Autodesk Inventor part; units mm, degrees
ref_plane "YZ Plane" through (0, 0, 0) normal (1, 0, 0) x (0, 1, 0)
ref_plane "XZ Plane" through (0, 0, 0) normal (0, 1, 0) x (-1, 0, 0)
ref_plane "XY Plane" through (0, 0, 0) normal (0, 0, 1) x (1, 0, 0)
sketch "Sketch1" plane through (0, 0, 0) normal (0, 1, 0) x (-1, 0, 0)
  line L0 (13.2677, 19.6408) -> (-12.1323, 19.6408)
  line L1 (-12.1323, 19.6408) -> (-12.1323, -18.4592)
  line L2 (-12.1323, -18.4592) -> (13.2677, -18.4592)
  line L3 (13.2677, -18.4592) -> (13.2677, 19.6408)
  point P0 (0, 0)
  dimension "d0" = 25.4
  dimension "d1" = 38.1
extrude "Extrusion1" add sketch "Sketch1" along normal blind 3.175
hole "Hole1" at (-9.6799, 3.175, 14.8783) direction (0, -1, 0) diameter 4.4958 depth 3.175
hole "Hole2" at (8.5446, 3.175, 14.8783) direction (0, -1, 0) diameter 4.4958 depth 3.175
hole "Hole3" at (-9.6799, 3.175, -13.6967) direction (0, -1, 0) diameter 4.4958 depth 3.175
hole "Hole4" at (8.5446, 3.175, -13.6967) direction (0, -1, 0) diameter 4.4958 depth 3.175
hole "Hole5" at (-0.5677, 3.175, -6.5466) direction (0, -1, 0) diameter 2.54 depth 3.175
hole "Hole6" at (-0.5677, 3.175, 7.7345) direction (0, -1, 0) diameter 2.54 depth 3.175
sketch "Sketch2" plane through (0, 3.175, 0) normal (0, 1, 0) x (1, 0, 0)
  circle A0 centre (0, 0) radius 3.175
  dimension "d58" = 6.35
extrude "Extrusion2" add sketch "Sketch2" along normal blind 304.8
sketch "Sketch3" plane through (0, 0, 0) normal (1, 0, 0) x (0, 1, 0)
  point P0 (0, 0)
properties part number "rotatable rod table"
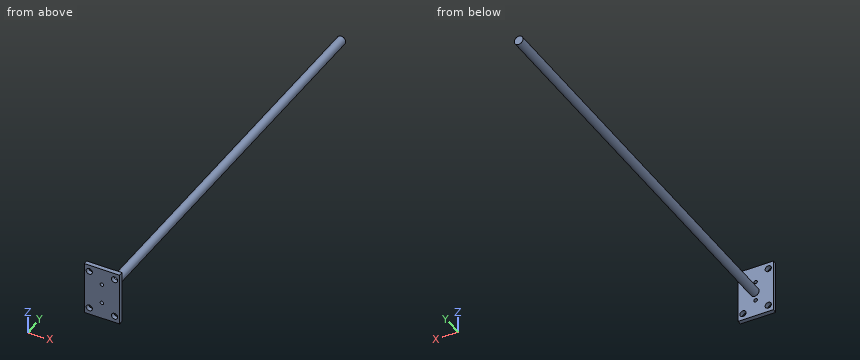
Model file for the job. Use its own axes, mm. Give positions to 0.01 mm unless a question says otherwise; leave off trailing zeros. Order: outer loops, then holes, each group sorted by start corner. A loop starts at its lowest first (then second) coordinate and runs counter-clockwise, first axis right, second up. Notation, with made-up numbers: (42.5, 33.5) - (92.5, 33.5) arc R21 ccw to (92.5, 41.5) - close; hole circle Ø5 at (49.25, -10). An arc over 180 degrees is marked (long way). Return JSON: item names as keys, results as strings.
1) Flat gauge pins, fed straight in: P1, Ø7.5, axis at x = -6.5, z = -5.5, coming from the +Y side (3 decimals); P2, Ø6, axis at y = 131, z = 1.5, coming from the -X side (3 decimals); P3, Ø7, axis at x = -9.68, z = -13.7, coming from the -Y side. Where does each tip first touch, or does it go through?
Geometry says:
{"P1": "y = 3.175", "P2": "x = -3.175", "P3": "y = 0"}
2) Probe line 1 (Y direction, x = -10.25, z = 17.5) (3 decimals); line 2 (Z direction, x = 0, y = 269) (3 decimals); line 3 (X direction, y = 177, z = 1). List the from-to ranges inside material, lowest first. Write a range as from..to.
Geometry says:
{"line 1": "0..3.175", "line 2": "-3.175..3.175", "line 3": "-3.01..3.01"}
3) Cut at A-A, the plane z = 0. Give the cut face in (x, y) (3 decimals), plus the area to 3 significant figures.
Geometry says:
{"outline": "(-13.268, 0) - (12.132, 0) - (12.132, 3.175) - (3.175, 3.175) - (3.175, 307.975) - (-3.175, 307.975) - (-3.175, 3.175) - (-13.268, 3.175) - close", "area": "2,020 mm²"}
4) Cut at B-B, the plane y = 247. Give the cut face in (x, z) (3 decimals).
Geometry says:
{"outline": "circle Ø6.35 at (0, 0)"}
